from build123d import *

# Parameters (mm, degrees)
BOSS_EXTRUDE1_DEPTH = 1.524
SKETCH2_W           = 1.524
SKETCH2_H           = 4.7498
CUT_EXTRUDE1_DEPTH  = 2.54


with BuildPart() as part:
    # Sketch1 → Boss-Extrude1 (new body)
    with BuildSketch(Plane.XY):
        with BuildLine():
            Line((-1.524, 17.137880282), (-1.524, 14.009051361))
            ThreePointArc((-1.524, 14.009051361), (-7.800379553, 17.247782791), (-14.842010982, 17.793446045))
            ThreePointArc((-14.842010982, 17.793446045), (-20.434373625, 26.496185152), (-22.17694037, 36.693030204))
            ThreePointArc((-22.17694037, 36.693030204), (-15.549040276, 33.631644025), (-8.706859323, 31.08493933))
            ThreePointArc((-8.706859323, 31.08493933), (-0.762, 29.81042814), (7.182859323, 31.08493933))
            ThreePointArc((7.182859323, 31.08493933), (14.025040276, 33.631644025), (20.65294037, 36.693030204))
            ThreePointArc((20.65294037, 36.693030204), (18.910373625, 26.496185152), (13.318010982, 17.793446045))
            ThreePointArc((13.318010982, 17.793446045), (6.276379553, 17.247782791), (0, 14.009051361))
            Line((0, 14.009051361), (0, 17.137880282))
            Line((0, 17.137880282), (-1.524, 17.137880282))
        make_face()
    extrude(amount=BOSS_EXTRUDE1_DEPTH)

    # Sketch2 → Cut-Extrude1 (cut)
    with BuildSketch(Plane.XY.offset(1.524)):
        with Locations((-11.049, 24.592780282)):
            Rectangle(SKETCH2_W, SKETCH2_H)
        with Locations((9.525, 24.592780282)):
            Rectangle(SKETCH2_W, SKETCH2_H)
    extrude(amount=-CUT_EXTRUDE1_DEPTH, mode=Mode.SUBTRACT)


solid = part.part
For this review, take the finished solid that the model builds, in its own axes (mm). A direction names the side the tool comes from. Round coordinates to 2 decimals unless told otherwise and drop trailing zeros. Loops run counter-clockwise (first coordinate to the right, second up) from the corner with the lowest first, then second, coordinate; pieces in that order, holes last. Notation, with made-up numbers: (-23, 80.25) - (5, 80.25) arc R18 cw to (5, 88.25) - close; hole circle Ø2 at (-17.75, 72). An arc over 180 degrees is marked (long way). One line per item, written item: value. Start each with the question number.
Item 1: For faces 1 (the flat face through (10.287, 25, 1)), 2 (the flat face through (-1.524, 16, 1)), 3 (the cylindrical face through (-15.64, 33.67, 0.75)), 4 (the flat face through (0, 26, 0)), list the 3-axis set-ups (+Z, -Z, +X, -X, +Y, -Y) from which the entire face can be reached by the end or side of a thin tool; tool diameter is ignored.
Item 2: Take a section at A-A (z = 0.85). Give the boundary of the cut face in (x, y), plus the area to 3 significant figures.
Item 3: Clearance check with flat-ended pins moving along their axes: pin 1 Ø0.8 at (y, z) = (15, 1) entering from +X; pin 2 Ø0.8 at (x, z) = (9.5, 1) entering from -Y; pin 3 Ø0.8 at (y, z) = (24, 1) entering from +X. State where each tip first meets the part, or that it passes through.
Item 4: The part is to be moulded in two halves that separate along X. For faces 5 (the flat face through (0, 26, 1.524)), 6 (the cylindrical face through (-20.38, 26.36, 0.75)), 7 (the cylindrical face through (-7.7, 17.22, 0.75)), say which applies: +X half, -X half, draft (parallel to the pull), parting line (faces both ways), or undercut.
Item 5: Take a section at C-C (y = 33). Give the boundary of the cut face in (x, z).
Item 6: For L1, parallel to X at y = 22.75, z = 0.8; L2, parallel to X at y = 26, z = 0.2; L3, parallel to Y at x = -0.5, z = 0.5, list the stretches that pass through material, from the lowest coordinate up.
Item 7: Take a section at D-D (x = -11). Give the boundary of the cut face in (y, z).
Item 8: Take a section at B-B (y = 23.5). Give the boundary of the cut face in (x, z).
Answer below:
1. face 1: +Z, -Z
1. face 2: +Z, -Z, -Y
1. face 3: +Z, -Z, +Y
1. face 4: -Z, +X, -X, +Y, -Y
2. outline: (-22.18, 36.69) arc R25.91 ccw to (-14.84, 17.79) arc R17.82 cw to (-1.52, 14.01) - (-1.52, 17.14) - (0, 17.14) - (0, 14.01) arc R17.82 cw to (13.32, 17.79) arc R25.91 ccw to (20.65, 36.69) arc R95.61 cw to (7.18, 31.08) arc R25.4 cw to (-8.71, 31.08) arc R95.61 cw to start; hole (-11.81, 22.22) - (-10.29, 22.22) - (-10.29, 26.97) - (-11.81, 26.97) - close; hole (8.76, 22.22) - (10.29, 22.22) - (10.29, 26.97) - (8.76, 26.97) - close
2. area: 554 mm2
3. pin 1: stops at x = 2
3. pin 2: stops at y = 17.81
3. pin 3: stops at x = 17.99
4. face 5: draft
4. face 6: -X half
4. face 7: undercut
5. outline: (-22.03, 0) - (-13.99, 0) - (-13.99, 1.52) - (-22.03, 1.52) - close; (12.47, 0) - (20.51, 0) - (20.51, 1.52) - (12.47, 1.52) - close
6. L1: x = -18.62 to -11.81, -10.29 to 8.76, 10.29 to 17.1
6. L2: x = -20.24 to -11.81, -10.29 to 8.76, 10.29 to 18.71
6. L3: y = 17.14 to 29.81
7. outline: (17.85, 0) - (22.22, 0) - (22.22, 1.52) - (17.85, 1.52) - close; (26.97, 0) - (31.87, 0) - (31.87, 1.52) - (26.97, 1.52) - close
8. outline: (-19.05, 0) - (-11.81, 0) - (-11.81, 1.52) - (-19.05, 1.52) - close; (-10.29, 0) - (8.76, 0) - (8.76, 1.52) - (-10.29, 1.52) - close; (10.29, 0) - (17.52, 0) - (17.52, 1.52) - (10.29, 1.52) - close
